The model under review builds one solid part; all positions refer to its coordinate system, in mm. Face numbers are marked on the shaded views. A direction names the side the tool comes from. Round coordinates to 2 decimals unless told otherwise and drop trailing zeros. Loops run counter-clockwise (first coordinate to the right, second up) from the corner with the lowest first, then second, coordinate; pieces in that order, holes last. Notation, with made-up numbers: M -39,-5 L 20,-5 A35 ccw 20,32 Z; hole C 1.25,23 d1. An arc over 180 degrees is marked long. Answer in a Markdown table with one row per item. Add a question column.
from build123d import *

# Parameters (mm, degrees)
SKETCH2_R           = 4.7
BOSS_EXTRUDE1_DEPTH = 45
SKETCH3_R           = 6.75
BOSS_EXTRUDE2_DEPTH = 2
CHAMFER1_SIZE       = 0.6


with BuildPart() as part:
    # Sketch2 → Boss-Extrude1 (new body)
    with BuildSketch(Plane(origin=(0, 0, 0), x_dir=(1, 0, 0), z_dir=(0, 1, 0))):
        Circle(SKETCH2_R)
    extrude(amount=BOSS_EXTRUDE1_DEPTH)

    # Sketch3 → Boss-Extrude2 (add)
    with BuildSketch(Plane(origin=(0, 45, 0), x_dir=(1, 0, 0), z_dir=(0, 1, 0))):
        Circle(SKETCH3_R)
    extrude(amount=-BOSS_EXTRUDE2_DEPTH)

    # Chamfer1
    chamfer1_edges = [part.edges().sort_by_distance(p)[0] for p in [
        (-4.7, 0, 0),
        (-6.75, 45, 0),
        (-6.75, 43, 0),
    ]]
    chamfer(chamfer1_edges, length=CHAMFER1_SIZE)


solid = part.part
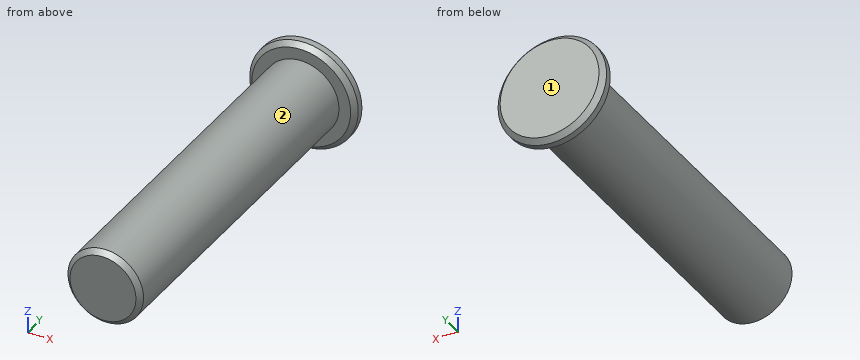
1. Take a section at C-C, the plane y = 34. State the section outline as (x, z) points, and give its area (3 significant figures).
2. For pin 1 Ø8 at (y, z) = (23.5, 3.5) entering from -X; pin 2 Ø8 at (x, y) = (-3.5, 7) entering from -Z; pin 3 Ø8 at (x, y) = (2.5, 18) entering from +Z, all flat-tipped, find the tip position at first contact; note any pin that passes through.
3. To check wall thickness, follow probe 1 along Y at (x, z) = (-4.5, 3); probe 2 along Z at (x, y) = (0, 40); probe 3 along Z at (x, y) = (2.5, 28.5). State the ranges of each line that lie inside material, in increasing order.
4. Take a section at B-B, the plane z = 0. State the section outline as (x, y) points, and give its area (3 significant figures).
5. Machinability: for the marked faces 1 and 2, which of the approach directions +Z, -Z, +X, -X, +Y, -Y give a long, thin tool a straight path to every point of the face, cutting with its end or side? Answer none if there is none.
6. Take a section at A-A, the plane x = 0. State the section outline as (y, z) points.
Check sheet entries:
| question | item | result |
|---|---|---|
| 1 | outline | C 0,0 d9.4 |
| 1 | area | 69.4 mm^2 |
| 2 | pin 1 | stops at x = -4.7 |
| 2 | pin 2 | stops at z = -4.7 |
| 2 | pin 3 | stops at z = 4.7 |
| 3 | probe 1 | y = 43 to 45 |
| 3 | probe 2 | z = -4.7 to 4.7 |
| 3 | probe 3 | z = -3.98 to 3.98 |
| 4 | outline | M -6.75,43.6 L -6.15,43 L -4.7,43 L -4.7,0.6 L -4.1,0 L 4.1,0 L 4.7,0.6 L 4.7,43 L 6.15,43 L 6.75,43.6 L 6.75,44.4 L 6.15,45 L -6.15,45 L -6.75,44.4 Z |
| 4 | area | 430 mm^2 |
| 5 | face 1 | +Z, -Z, +X, -X, +Y |
| 5 | face 2 | -Y |
| 6 | outline | M 0,-4.1 L 0.6,-4.7 L 43,-4.7 L 43,-6.15 L 43.6,-6.75 L 44.4,-6.75 L 45,-6.15 L 45,6.15 L 44.4,6.75 L 43.6,6.75 L 43,6.15 L 43,4.7 L 0.6,4.7 L 0,4.1 Z |
